from build123d import *

# Parameters (mm, degrees)
F0_W          = 5.2
F0_H          = 2.2
F1_DEPTH      = 12.5
F2_W          = 5.2
F2_H          = 4
F3_DEPTH      = 3.5
F5_DEPTH      = 10.5
F5_DEPTH_BACK = 5.5
F7_DEPTH      = 5
F8_R          = 1.99999


# Not quite as in the source:
# - a fillet or chamfer is up to 0.001 mm smaller than in the source, because OpenCascade refuses the exact size


with BuildPart() as f1:
    # F0 (on Front) → F1 (new body)
    with BuildSketch(Plane.XZ):
        with Locations((-2.6, 1.1)):
            Rectangle(F0_W, F0_H)
    extrude(amount=-F1_DEPTH)

    # F2 (on face) → F3 (join)
    with BuildSketch(Plane.XY.offset(2.2)):
        with Locations((-2.6, 10.5)):
            Rectangle(F2_W, F2_H)
    extrude(amount=F3_DEPTH)

    # F4 (on face) → F5 (join, two sides)
    with BuildSketch(Plane.YZ) as f5_sk:
        Polygon((12.5, 0), (12.5, 5.7), (8.5, 5.7), (8.5, 2.2), (8.5, 0), align=None)
    extrude(amount=-F5_DEPTH)
    extrude(f5_sk.sketch, amount=F5_DEPTH_BACK)

    # F6 (on face) → F7 (cut)
    with BuildSketch(Plane.XY.offset(5.7)):
        with BuildLine():
            Line((-9.2, 10.5), (-8, 10.5))
            Line((-8, 10.5), (-6.8, 10.5))
            ThreePointArc((-6.8, 10.5), (-8, 11.7), (-9.2, 10.5))
        make_face()
        with BuildLine():
            Line((-6.8, 10.5), (-8, 10.5))
            Line((-8, 10.5), (-9.2, 10.5))
            ThreePointArc((-9.2, 10.5), (-8, 9.3), (-6.8, 10.5))
        make_face()
        with BuildLine():
            Line((3, 10.5), (1.8, 10.5))
            ThreePointArc((1.8, 10.5), (3, 9.3), (4.2, 10.5))
            Line((4.2, 10.5), (3, 10.5))
        make_face()
        with BuildLine():
            ThreePointArc((4.2, 10.5), (3, 11.7), (1.8, 10.5))
            Line((1.8, 10.5), (3, 10.5))
            Line((3, 10.5), (4.2, 10.5))
        make_face()
    extrude(amount=-F7_DEPTH, mode=Mode.SUBTRACT)

    # F8 (radius 2 in the source; OpenCascade refuses exactly that, so slightly less here)
    f8_edges = [f1.edges().sort_by_distance(p)[0] for p in [
        (5.5, 8.5, 2.85),
        (5.5, 12.5, 2.85),
        (-10.5, 12.5, 2.85),
        (-10.5, 8.5, 2.85),
    ]]
    fillet(f8_edges, radius=F8_R)


solid = f1.part
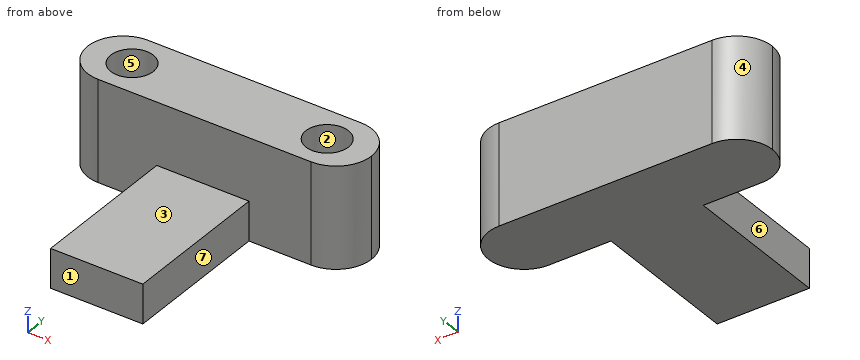
Geometry check sheet. Reference: the model listing, model coordinates, mm. Face numbers are marked on the shaded views. A direction names the side the tool comes from. Round coordinates to 2 decimals unless told otherwise and drop trailing zeros. Loops run counter-clockwise (first coordinate to the right, second up) from the corner with the lowest first, then second, coordinate; pieces in that order, holes last. Notation, with made-up numbers: (58.5, 44.25) -> (116.5, 44.25) arc R28 ccw to (116.5, 64.25) -> close; hole circle Ø1 at (46, 7). An arc over 180 degrees is marked (long way). Answer as a JSON object with one key per item and string values. Group by question number.
Item 1: Cross-section at C-C, the plane y = 7.75. Record the cut outline in (x, z).
Item 2: Thickness scan on line 1 along X through (y, z) = (10, 2.5); line 2 along Y through (x, z) = (-2, 5.35); line 3 along Z through (x, y) = (-0.5, 4.75). Record the ranges inside material, lowest first.
Item 3: Depth check by flat-ended pin: pin 1 Ø1.2 at (x, y) = (3.5, 10.5) entering from +Z; pin 2 Ø0.7 at (y, z) = (4, 1) entering from -X; pin 3 Ø4 at (x, y) = (-2.5, 3.5) entering from +Z. Enter the tip coordinate at first touch or a pass-through.
Item 4: Cross-section at B-B, the plane x = 3. Record the cut outline in (y, z).
Item 5: Release check for a two-part mould opening along Y. For the marked faces 1, 2 and 3 record: pulls with the +Y half, pulls with the -Y half, needs draft (parallel to the pull), parting line crosses it, or undercut.
Item 6: Cross-section at A-A, the plane z = 3.5. Count the separate pieces of the cut face and the enclosed holes in it, plus the area to 3 significant figures.
Item 7: Set-up check for the marked faces 4, 5, 6 and 7: record each of +Z, -Z, +X, -X, +Y, -Y from which the full face is reachable in a straight line by a thin tool's end or side.
Determined:
{
 "1": {"outline": "(-5.2, 0) -> (0, 0) -> (0, 2.2) -> (-5.2, 2.2) -> close"},
 "2": {"line 1": "x = -10.44 to -9.09, -6.91 to 1.91, 4.09 to 5.44", "line 2": "y = 8.5 to 12.5", "line 3": "z = 0 to 2.2"},
 "3": {"pin 1": "stops at z = 0.7", "pin 2": "stops at x = -5.2", "pin 3": "stops at z = 2.2"},
 "4": {"outline": "(8.5, 0) -> (12.5, 0) -> (12.5, 5.7) -> (11.7, 5.7) -> (11.7, 0.7) -> (9.3, 0.7) -> (9.3, 5.7) -> (8.5, 5.7) -> close"},
 "5": {"face 1": "pulls with the -Y half", "face 2": "undercut", "face 3": "needs draft"},
 "6": {"separate pieces": "1", "enclosed holes": "2", "area": "51.5 mm²"},
 "7": {"face 4": "+Z, -Z, -X, +Y", "face 5": "+Z", "face 6": "+Z, -Z, -X, -Y", "face 7": "+Z, -Z, +X, -Y"}
}
